Here's how the part is built. I have some questions about the finished solid (model axes, mm). Give positions to 0.01 mm unless a question says otherwise; leave off trailing zeros. Write each loop counter-clockwise with the first axis right and the second up, starting at its lowest first coordinate (ties: lowest second). Pieces come first, ordered by that corner, then holes. Notation, with made-up numbers: (-3, 64) -> (24, 64) arc R14 ccw to (24, 79) -> close; hole circle Ø1 at (0, -29). An arc over 180 degrees is marked (long way). Return JSON: item names as keys, results as strings.
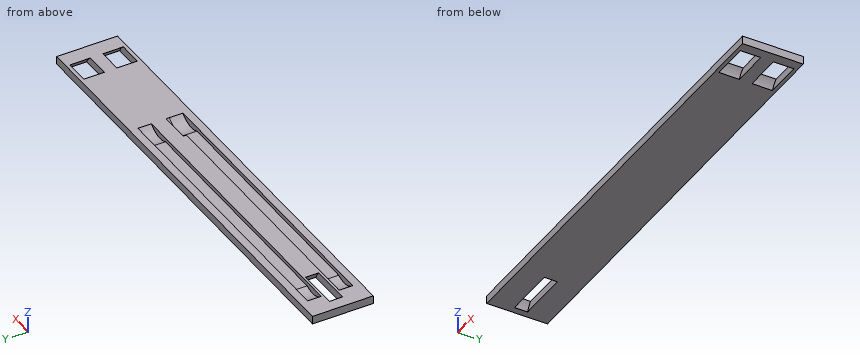
from build123d import *

# Parameters (mm, degrees)
CROQUIS1_W              = 985
CROQUIS1_H              = 135
SALIENTE_EXTRUIR1_DEPTH = 18
CROQUIS2_R              = 45
CORTAR_EXTRUIR1_DEPTH   = 45.5
CROQUIS4_R              = 62.2
CORTAR_EXTRUIR2_DEPTH   = 14.5
CORTAR_EXTRUIR3_DEPTH   = 15
CROQUIS7_R              = 46
CORTAR_EXTRUIR4_DEPTH   = 7


with BuildPart() as part:
    # Croquis1 → Saliente-Extruir1 (new body)
    with BuildSketch(Plane.XY):
        with Locations((492.5, 67.5)):
            Rectangle(CROQUIS1_W, CROQUIS1_H)
    extrude(amount=SALIENTE_EXTRUIR1_DEPTH)

    # Croquis2 → Cortar-Extruir1 (cut)
    with BuildSketch(Plane(origin=(0, 8, 0), x_dir=(-1, 0, 0), z_dir=(0, -1, 0))):
        with Locations((-921.5, 18)):
            Circle(CROQUIS2_R)
    cortar_extruir1 = extrude(amount=-CORTAR_EXTRUIR1_DEPTH, mode=Mode.SUBTRACT)

    # Simetría1: Cortar-Extruir1 across plane
    add(cortar_extruir1.mirror(Plane.ZX.offset(67.5)), mode=Mode.SUBTRACT)

    # Croquis4 → Cortar-Extruir2 (cut, symmetric)
    with BuildSketch(Plane(origin=(0, 67.5, 0), x_dir=(1, 0, 0), z_dir=(0, 1, 0))):
        with Locations((72.2, 24.2)):
            Circle(CROQUIS4_R)
    extrude(amount=CORTAR_EXTRUIR2_DEPTH, both=True, mode=Mode.SUBTRACT)

    # Croquis5 → Cortar-Extruir3 (cut, symmetric)
    with BuildSketch(Plane(origin=(0, 102.5, 0), x_dir=(1, 0, 0), z_dir=(0, 1, 0))):
        with BuildLine():
            Line((102.856653615, -9), (649.052499818, -9))
            ThreePointArc((649.052499818, -9), (677.48487297, -4.628109214), (702.954576716, -18))
            Line((702.954576716, -18), (48.954576716, -18))
            ThreePointArc((48.954576716, -18), (74.424280462, -4.628109214), (102.856653615, -9))
        make_face()
    cortar_extruir3 = extrude(amount=CORTAR_EXTRUIR3_DEPTH, both=True, mode=Mode.SUBTRACT)

    # Simetría5: Cortar-Extruir3 across plane
    add(cortar_extruir3.mirror(Plane.ZX.offset(67.5)), mode=Mode.SUBTRACT)

    # Croquis7 → Cortar-Extruir4 (cut)
    with BuildSketch(Plane.XZ.offset(-47.5)):
        with Locations((669.909153433, 50)):
            Circle(CROQUIS7_R)
    extrude(amount=-CORTAR_EXTRUIR4_DEPTH, mode=Mode.SUBTRACT)


solid = part.part
1. Suppose I cut it at C-C, the plane z = 12.5. List the corners of the cut face in (x, y) for me, and give its area (3 significant figures).
Taken from the geometry:
{"outline": "(0, 0) -> (985, 0) -> (985, 135) -> (0, 135) -> close; hole (21.98, 53) -> (122.42, 53) -> (122.42, 82) -> (21.98, 82) -> close; hole (55.36, 17.5) -> (696.55, 17.5) -> (696.55, 54.5) -> (643.27, 54.5) -> (643.27, 47.5) -> (55.36, 47.5) -> close; hole (55.36, 87.5) -> (696.55, 87.5) -> (696.55, 117.5) -> (55.36, 117.5) -> close; hole (888.41, 8) -> (954.59, 8) -> (954.59, 53.5) -> (888.41, 53.5) -> close; hole (888.41, 81.5) -> (954.59, 81.5) -> (954.59, 127) -> (888.41, 127) -> close", "area": "85,200 mm²"}
2. For pin 1 Ø9 at (x, y) = (323, 33) entering from +Z, with a flat end and sliding along its axis, tell me the tip position at first contact or that it passes through.
Taken from the geometry:
{"pin 1": "stops at z = 9"}
3. Suppose I cut it at A-A, the plane y = 62.5. List the corners of the cut face in (x, z) for me, and give its area (3 significant figures).
Taken from the geometry:
{"outline": "(0, 0) -> (14.9, 0) arc R62.2 cw to (26.51, 18) -> (0, 18) -> close; (117.89, 18) arc R62.2 cw to (129.5, 0) -> (985, 0) -> (985, 18) -> close", "area": "15,800 mm²"}
4. Suppose I cut it at D-D, the plane y = 102.5. List the corners of the cut face in (x, z) for me.
Taken from the geometry:
{"outline": "(0, 0) -> (880.26, 0) arc R45 cw to (894.5, 18) -> (702.95, 18) arc R46 cw to (649.05, 9) -> (102.86, 9) arc R46 cw to (48.95, 18) -> (0, 18) -> close; (948.5, 18) arc R45 cw to (962.74, 0) -> (985, 0) -> (985, 18) -> close"}
5. If I drill on line 1 (Y direction, x = 259, z = 17.25); line 2 (Y direction, x = 659, z = 7.5); line 3 (X direction, y = 112, z = 15.25), over which ranges is the centre line in solid material (lowest first)? Write a range as [from, to].
Taken from the geometry:
{"line 1": "y = [0, 17.5], [47.5, 87.5], [117.5, 135]", "line 2": "y = [0, 17.5], [54.5, 87.5], [117.5, 135]", "line 3": "x = [0, 51.86], [700.05, 891.18], [951.82, 985]"}
6. Suppose I cut it at B-B, the plane x = 575. List the corners of the cut face in (y, z) for me.
Taken from the geometry:
{"outline": "(0, 0) -> (135, 0) -> (135, 18) -> (117.5, 18) -> (117.5, 9) -> (87.5, 9) -> (87.5, 18) -> (47.5, 18) -> (47.5, 9) -> (17.5, 9) -> (17.5, 18) -> (0, 18) -> close"}
